from build123d import *

# Parameters (mm, degrees)
BOSS_EXTRUDE1_START          = -25.4
BOSS_EXTRUDE1_OUTLINE_W      = 63.5
BOSS_EXTRUDE1_OUTLINE_H      = 31.75
BOSS_EXTRUDE1_DEPTH          = 50.8
SKETCH2_W                    = 12.7
SKETCH2_H                    = 29.21
CUT_EXTRUDE1_DEPTH           = 25.4
SKETCH3_W                    = 12.7
SKETCH3_H                    = 29.21
CUT_EXTRUDE2_DEPTH           = 25.4
SKETCH4_W                    = 23.809600622
SKETCH4_H                    = 23.809600622
CUT_EXTRUDE3_DEPTH           = 3.25
SKETCH5_W                    = 12.108
SKETCH5_H                    = 47.55
F_2_0_2_DIAMETER_HOLE1_D     = 2
F_2_0_2_DIAMETER_HOLE1_DEPTH = 2.54
M7_CLEARANCE_HOLE1_D         = 7.508
M7_CLEARANCE_HOLE1_DEPTH     = 31.75
FILLET1_R                    = 5.08


with BuildPart() as part:
    # Boss-Extrude1: read off the stored shape, not the designer's step
    # Boss-Extrude1 outline → Boss-Extrude1 (new body)
    with BuildSketch(Plane.XZ.offset(25.4).offset(BOSS_EXTRUDE1_START)):
        Rectangle(BOSS_EXTRUDE1_OUTLINE_W, BOSS_EXTRUDE1_OUTLINE_H)
    extrude(amount=BOSS_EXTRUDE1_DEPTH)

    # Sketch2 → Cut-Extrude1 (cut)
    with BuildSketch(Plane(origin=(0, 0, 0), x_dir=(-1, 0, 0), z_dir=(0, 1, 0))):
        with Locations((-25.4, 1.27)):
            Rectangle(SKETCH2_W, SKETCH2_H)
    extrude(amount=-CUT_EXTRUDE1_DEPTH, mode=Mode.SUBTRACT)

    # Sketch3 → Cut-Extrude2 (cut)
    with BuildSketch(Plane(origin=(0, 0, 0), x_dir=(-1, 0, 0), z_dir=(0, 1, 0))):
        with Locations((25.4, 1.27)):
            Rectangle(SKETCH3_W, SKETCH3_H)
    extrude(amount=-CUT_EXTRUDE2_DEPTH, mode=Mode.SUBTRACT)

    # Sketch4 → Cut-Extrude3 (cut)
    with BuildSketch(Plane(origin=(0, 0, 0), x_dir=(-1, 0, 0), z_dir=(0, 1, 0))):
        Rectangle(SKETCH4_W, SKETCH4_H)
    extrude(amount=-CUT_EXTRUDE3_DEPTH, mode=Mode.SUBTRACT)

    # Sketch5 → M22 Clearance Hole1 (revolve, cut)
    with BuildSketch(Plane(origin=(0, -3.25, 0), x_dir=(0, 0, 1), z_dir=(1, 0, 0))):
        with Locations((6.054, 23.775)):
            Rectangle(SKETCH5_W, SKETCH5_H)
    revolve(axis=Axis((0, 3.1, 0), (0, -1, 0)), mode=Mode.SUBTRACT)

    # Ø2.0 (2) Diameter Hole1
    with Locations(Plane(origin=(0, 0, 0), x_dir=(1, 0, 0), z_dir=(0, 1, 0))):
        with Locations((14.5034, 0), (-14.5034, 0)):
            Hole(F_2_0_2_DIAMETER_HOLE1_D / 2, depth=F_2_0_2_DIAMETER_HOLE1_DEPTH)

    # M7 Clearance Hole1
    with Locations(Plane(origin=(0, 0, -15.875), x_dir=(-1, 0, 0), z_dir=(0, 0, -1))):
        with Locations((25.412960945, -12.423554609), (-25.412960945, -12.423554609)):
            Hole(M7_CLEARANCE_HOLE1_D / 2, depth=M7_CLEARANCE_HOLE1_DEPTH)

    # Fillet1
    fillet1_edges = [part.edges().sort_by_distance(p)[0] for p in [
        (19.05, -12.7, 15.875),
        (-19.05, -12.7, 15.875),
        (-31.75, 0, -14.605),
        (31.75, 0, -14.605),
    ]]
    fillet(fillet1_edges, radius=FILLET1_R)


solid = part.part
Can you work these out from the model? Positions are in its coordinate system, mm. A direction names the side the tool comes from. Round coordinates to 2 decimals unless told otherwise and drop trailing zeros. Order: outer loops, then holes, each group sorted by start corner. A loop starts at its lowest first (then second) coordinate and runs counter-clockwise, first axis right, second up. Notation, with made-up numbers: (7.5, 4) -> (44.5, 4) arc R27 ccw to (44.5, 37) -> close; hole circle Ø5 at (11, 40.5). An arc over 180 degrees is marked (long way). Write each question's results on one line, items separated by ' | '. Start each with the question number.
Item 1: Thinking about a two-plate mould opening in Z: for faces 4 (the flat face through (0, -31, 15.875)), 5 (the flat face through (-14, -2.54, 0)), 6 (the cylindrical face through (-26.227, -16.088, -14.587)), which applies, +Z half, -Z half, draft (parallel to the pull), parting line (faces both ways), or undercut?
Item 2: If we section it at D-D, the plane y = -46: Write out the boundary of the cut face in (x, z) (3 decimals).
Item 3: Please list where these lines run through material, in increasing order: L1, parallel to Z at x = 0, y = -25 (3 decimals); L2, parallel to X at y = -33, z = 0.5; L3, parallel to X at y = -3, z = 2.5.
Item 4: Which directions (+Z, -Z, +X, -X, +Y, -Y) give clear straight access to the entire face, cutting with the end or side of a thin tool? Please do faces 1 (the flat face through (-22, -15, -13.335)), 2 (the cylindrical face through (17.52, -12.88, 14.43)), 3 (the cylindrical face through (13.55, -1.29, -0.3)).
Item 5: If we section it at C-C, the plane x = 0: Write out the boundary of the cut face in (y, z) (3 decimals).
Item 6: If we section it at B-B, the plane z = 0: Write out the boundary of the cut face in (x, y).
Item 7: If we section it at A-A, the plane y = -24: Write out the boundary of the cut face in (x, z) (3 decimals), then the cut area to 3 significant figures.
Item 8: Will these pins go through, and if not, where does the flat tip stop? pin 1 (1.6 mm diameter, centred on x = -14.5, z = 0, fed in from +Y); pin 2 (3 mm diameter, centred on x = -6.5, z = 8, fed in from +Y); pin 3 (3 mm diameter, centred on x = 18.5, z = -7.5, fed in from +Y); pin 4 (1.6 mm diameter, centred on y = -1.5, z = 4.5, fed in from +X).
Results:
1) face 4: +Z half | face 5: undercut | face 6: draft
2) outline: (-31.75, -15.875) -> (31.75, -15.875) -> (31.75, 15.875) -> (-31.75, 15.875) -> close; hole circle Ø24.216 at (0, 0)
3) L1: z = -15.875 to -12.108, 12.108 to 15.875 | L2: x = -31.75 to -12.1, 12.1 to 31.75 | L3: x = -19.05 to -11.9, 11.9 to 19.05
4) face 1: +Z, -X, +Y | face 2: +Z, +X, +Y | face 3: +Y
5) outline: (-50.8, -15.875) -> (0, -15.875) -> (0, -11.905) -> (-3.25, -11.905) -> (-3.25, -12.108) -> (-50.8, -12.108) -> close; (-50.8, 12.108) -> (-3.25, 12.108) -> (-3.25, 11.905) -> (0, 11.905) -> (0, 15.875) -> (-50.8, 15.875) -> close
6) outline: (-31.75, -50.8) -> (-12.11, -50.8) -> (-12.11, -3.25) -> (-11.9, -3.25) -> (-11.9, 0) -> (-13.5, 0) -> (-13.5, -2.54) -> (-15.5, -2.54) -> (-15.5, 0) -> (-19.05, 0) -> (-19.05, -25.4) -> (-31.75, -25.4) -> close; (11.9, -3.25) -> (12.11, -3.25) -> (12.11, -50.8) -> (31.75, -50.8) -> (31.75, -25.4) -> (19.05, -25.4) -> (19.05, 0) -> (15.5, 0) -> (15.5, -2.54) -> (13.5, -2.54) -> (13.5, 0) -> (11.9, 0) -> close
7) outline: (-31.75, -15.875) -> (31.75, -15.875) -> (31.75, -13.335) -> (19.05, -13.335) -> (19.05, 10.795) arc R5.08 ccw to (13.97, 15.875) -> (-13.97, 15.875) arc R5.08 ccw to (-19.05, 10.795) -> (-19.05, -13.335) -> (-31.75, -13.335) -> close; hole circle Ø24.216 at (0, 0) | area: 803 mm2
8) pin 1: stops at y = -2.54 | pin 2: passes through | pin 3: stops at y = 0 | pin 4: stops at x = 19.05
